Could you check a few things on this drawing? It's one solid part, dimensions in mm from its lowest x, y, z. A direction names the side the tool comes from. Give positions to 0.01 mm unless a question says otherwise; leave off trailing zeros. Order: outer loops, then holes, each group sorted by start corner. A loop starts at its lowest first (then second) coordinate and runs counter-clockwise, first axis right, second up. Notation, with made-up numbers: M 11.5,-17.75 L 29.5,-17.75 A7 ccw 29.5,-10.75 Z; hole C 43,79.5 d11. An arc over 180 degrees is marked long. Return JSON: item names as keys, results as strings. Group by question number.
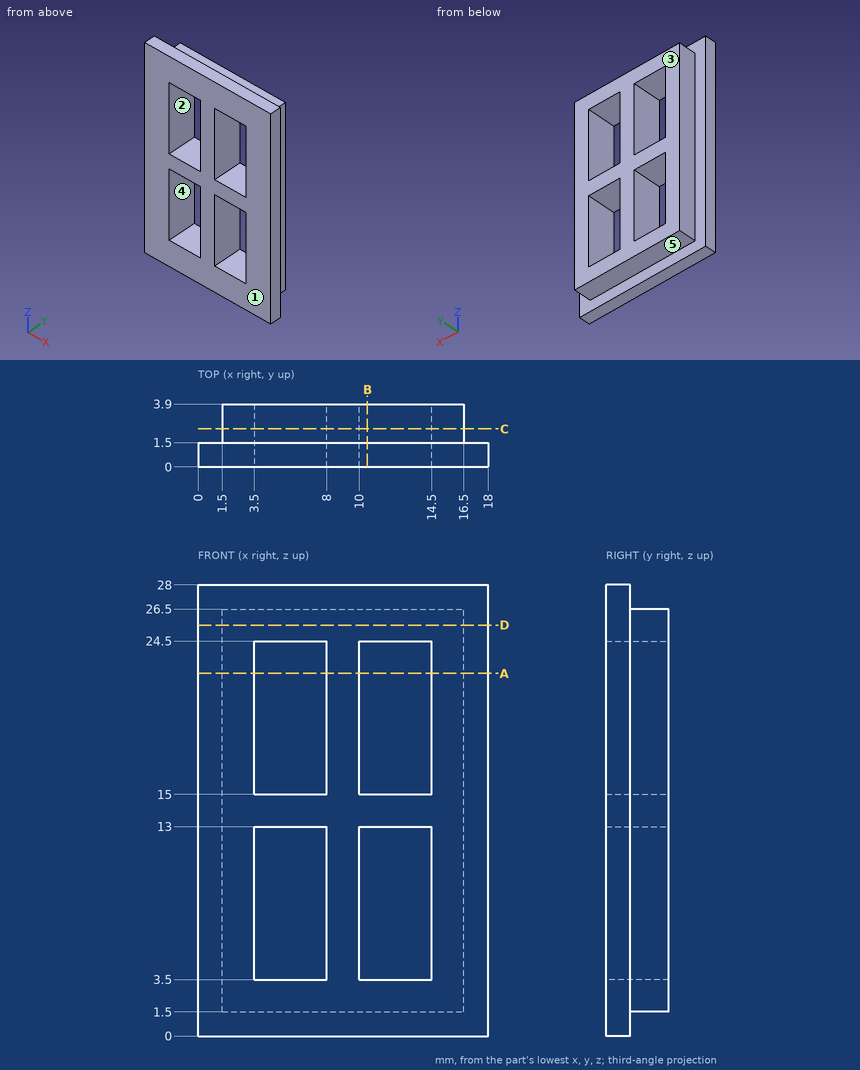
1. If we mould it in two halves opening along X, with no side actions, what happens to the marked faces 1 and 2? For each: pulls with the +X half, pulls with the -X half, needs draft (parallel to the pull), parting line crosses it, or undercut.
2. Which directions (+Z, -Z, +X, -X, +Y, -Y) give clear straight access to the entire face, cutting with the end or side of a thin tool? Please do the marked faces 3, 4 and 5.
3. Imagine slicing it at B-B, the plane x = 10.5. Please give me the cut outline in (y, z).
4. Imagine slicing it at D-D, the plane z = 25.5. Please give me the cut outline in (x, y), plus the area to 3 significant figures.
5. I need wall thicknesses on L1, parallel to X at y = 2.95, z = 15.5; L2, parallel to X at y = 0.7, z = 21.25; L3, parallel to Z at x = 6.25, y = 3.4. Which ranges of each line are inside material? Lowest first, please. Write a range as from..to.
6. Imagine slicing it at A-A, the plane z = 22.5. Please give me the cut outline in (x, y).
7. Imagine slicing it at C-C, the plane y = 2.35. Please give me the cut outline in (x, z), plus the area to 3 significant figures.
8. For pin 1 (1.9 mm diameter, centred on y = 2, z = 15, fed in from -X); pin 2 (2 mm diameter, centred on x = 15, y = 3.5, fed in from +Z); pin 3 (1.5 mm diameter, centred on x = 4.5, y = 3, fed in from -Z); pin 4 (1.2 mm diameter, centred on y = 2.5, z = 21.5, fed in from +X), each with a flat end and sliding along its axis, tell me the tip position at first contact or that it passes through.
Values:
{
 "1": {"face 1": "needs draft", "face 2": "undercut"},
 "2": {"face 3": "+Z, -Z, +X, -X, +Y", "face 4": "+Y, -Y", "face 5": "-Z, +X, -X, +Y"},
 "3": {"outline": "M 0,0 L 1.5,0 L 1.5,1.5 L 3.9,1.5 L 3.9,3.5 L 0,3.5 Z; M 0,13 L 3.9,13 L 3.9,15 L 0,15 Z; M 0,24.5 L 3.9,24.5 L 3.9,26.5 L 1.5,26.5 L 1.5,28 L 0,28 Z"},
 "4": {"outline": "M 0,0 L 18,0 L 18,1.5 L 16.5,1.5 L 16.5,3.9 L 1.5,3.9 L 1.5,1.5 L 0,1.5 Z", "area": "63.0 mm²"},
 "5": {"L1": "x = 1.5..3.5, 8..10, 14.5..16.5", "L2": "x = 0..3.5, 8..10, 14.5..18", "L3": "z = 1.5..3.5, 13..15, 24.5..26.5"},
 "6": {"outline": "M 0,0 L 3.5,0 L 3.5,3.9 L 1.5,3.9 L 1.5,1.5 L 0,1.5 Z; M 8,0 L 10,0 L 10,3.9 L 8,3.9 Z; M 14.5,0 L 18,0 L 18,1.5 L 16.5,1.5 L 16.5,3.9 L 14.5,3.9 Z"},
 "7": {"outline": "M 1.5,1.5 L 16.5,1.5 L 16.5,26.5 L 1.5,26.5 Z; hole M 3.5,3.5 L 8,3.5 L 8,13 L 3.5,13 Z; hole M 3.5,15 L 8,15 L 8,24.5 L 3.5,24.5 Z; hole M 10,3.5 L 14.5,3.5 L 14.5,13 L 10,13 Z; hole M 10,15 L 14.5,15 L 14.5,24.5 L 10,24.5 Z", "area": "204 mm²"},
 "8": {"pin 1": "stops at x = 0", "pin 2": "stops at z = 26.5", "pin 3": "stops at z = 1.5", "pin 4": "stops at x = 16.5"}
}
